Work out the finished part from the listing and answer in its coordinate system (mm). A direction names the side the tool comes from. Coordinates: 2 decimals unless noted, no trailing zeros. Order: outer loops, then holes, each group sorted by start corner. A loop starts at its lowest first (then second) coordinate and runs counter-clockwise, first axis right, second up. Notation, with made-up numbers: M 59,-22 L 82,-22 A6 cw 82,-13 Z; hole C 57.25,11 d11. An arc over 180 degrees is marked long. Use a Markdown table: item, result.
from build123d import *

# Parameters (mm, degrees)
SKETCH1_W           = 13
SKETCH1_H           = 30
BOSS_EXTRUDE1_DEPTH = 15
SKETCH2_W           = 13
SKETCH2_H           = 3
BOSS_EXTRUDE2_DEPTH = 10
SKETCH3_R           = 1.05
CUT_EXTRUDE1_DEPTH  = 52.833163371


with BuildPart() as part:
    # Sketch1 → Boss-Extrude1 (new body)
    with BuildSketch(Plane(origin=(0, 0, 0), x_dir=(1, 0, 0), z_dir=(0, 1, 0))):
        with Locations((-30.005846449, -1.517902626)):
            Rectangle(SKETCH1_W, SKETCH1_H)
    extrude(amount=BOSS_EXTRUDE1_DEPTH)

    # Sketch2 → Boss-Extrude2 (add)
    with BuildSketch(Plane(origin=(0, 15, 0), x_dir=(1, 0, 0), z_dir=(0, 1, 0))):
        with Locations((-30.005846449, -15.017902626)):
            Rectangle(SKETCH2_W, SKETCH2_H)
    extrude(amount=BOSS_EXTRUDE2_DEPTH)

    # Sketch3 → Cut-Extrude1 (cut, through all)
    with BuildSketch(Plane(origin=(0, 0, 13.517902626), x_dir=(-1, 0, 0), z_dir=(0, 0, -1))):
        with Locations((30.005846449, 20)):
            Circle(SKETCH3_R)
    extrude(amount=-CUT_EXTRUDE1_DEPTH, mode=Mode.SUBTRACT)


solid = part.part
(1) Determine the mould class of faces 1 (the cylindrical face through (-30.976, 19.598, 14.997)), 2 (the flat face through (-23.506, 7, 2)), 3 (the flat face through (-30, 0, 1)) for opening direction X: pulls with the +X half, pulls with the -X half, needs draft (parallel to the pull), parting line crosses it, or undercut.
Conclusion:
| item | result |
|---|---|
| face 1 | undercut |
| face 2 | pulls with the +X half |
| face 3 | needs draft |
(2) A cutting plane is placed at C-C (z = -11.5). Determine the outline of the cut face in (x, y).
Conclusion:
| item | result |
|---|---|
| outline | M -36.51,0 L -23.51,0 L -23.51,15 L -36.51,15 Z |
(3) Straight lines are drawn through the part: L1, parallel to Y at x = -27, z = 4.75; L2, parallel to Z at x = -32.5, y = 22.75. For each, find the intervals that lie inside material, in ascending order.
Conclusion:
| item | result |
|---|---|
| L1 | 0 to 15 |
| L2 | 13.52 to 16.52 |
(4) A cutting plane is placed at A-A (y = 20). Determine the outline of the cut face in (x, z).
Conclusion:
| item | result |
|---|---|
| outline | M -36.51,13.52 L -31.06,13.52 L -31.06,16.52 L -36.51,16.52 Z; M -28.96,13.52 L -23.51,13.52 L -23.51,16.52 L -28.96,16.52 Z |
(5) A cutting plane is placed at B-B (x = -30). Determine the outline of the cut face in (y, z), then the cut area to 3 significant figures.
Conclusion:
| item | result |
|---|---|
| outline | M 0,-13.48 L 15,-13.48 L 15,13.52 L 18.95,13.52 L 18.95,16.52 L 0,16.52 Z; M 21.05,13.52 L 25,13.52 L 25,16.52 L 21.05,16.52 Z |
| area | 474 mm2 |
(6) Which of the six approach directions +Z, -Z, +X, -X, +Y, -Y give full straight-line access (tool end or side, diameter ignored) to faces 4 (the flat face through (-30, 12, 16.518)), 5 (the flat face through (-30, 15, 0))?
Conclusion:
| item | result |
|---|---|
| face 4 | +Z, +X, -X, +Y, -Y |
| face 5 | -Z, +X, -X, +Y |
(7) A cutting plane is placed at D-D (x = -28). Determine the outline of the cut face in (y, z), then the cut area to 3 significant figures.
Conclusion:
| item | result |
|---|---|
| outline | M 0,-13.48 L 15,-13.48 L 15,13.52 L 25,13.52 L 25,16.52 L 0,16.52 Z |
| area | 480 mm2 |
